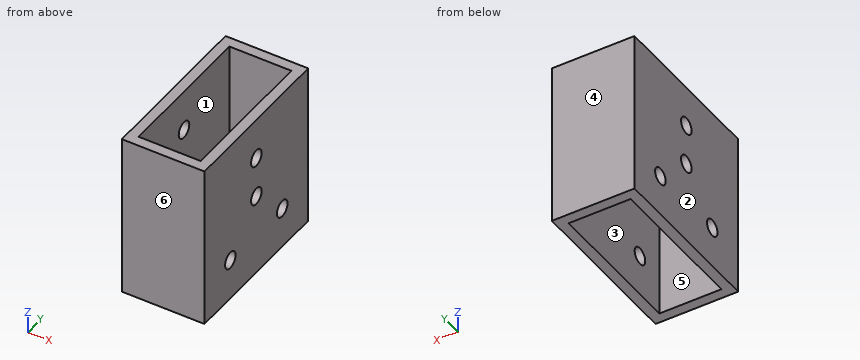
Autodesk Inventor part; units mm, degrees
ref_plane "YZ Plane" through (0, 0, 0) normal (1, 0, 0) x (0, 1, 0)
ref_plane "XZ Plane" through (0, 0, 0) normal (0, 1, 0) x (-1, 0, 0)
ref_plane "XY Plane" through (0, 0, 0) normal (0, 0, 1) x (1, 0, 0)
sketch "Sketch1" plane through (0, 0, 0) normal (0, 0, 1) x (1, 0, 0)
  line L0 (0, 0) -> (25.4, 0)
  line L1 (25.4, 0) -> (25.4, 50.8)
  line L2 (25.4, 50.8) -> (0, 50.8)
  line L3 (0, 50.8) -> (0, 0)
  line L4 (3.175, 47.625) -> (22.225, 47.625)
  line L5 (22.225, 47.625) -> (22.225, 3.175)
  line L6 (22.225, 3.175) -> (3.175, 3.175)
  line L7 (3.175, 3.175) -> (3.175, 47.625)
  dimension "d0" = 25.4
  dimension "d1" = 50.8
  dimension "d2" = 3.175
extrude "Extrusion1" add sketch "Sketch1" along normal blind 50.8
sketch "Sketch2" plane through (25.4, 0, 0) normal (1, 0, 0) x (0, 0, -1)
  line L0 (0, 50.8) -> (0, 0) construction
  line L1 (0, 0) -> (-12.7, 0) construction
  line L2 (0, 0) -> (-50.8, 0) construction
  line L3 (-12.7, 0) -> (-12.7, 12.7) construction
  line L4 (-12.7, 12.7) -> (-12.7, 38.1) construction
  circle A0 centre (-12.7, 12.7) radius 2.5797
  circle A1 centre (-12.7, 38.1) radius 2.5797
  dimension "d5" = 12.7
  dimension "d6" = 12.7
  dimension "d7" = 25.4
  dimension "d8" = 5.1594
extrude "Extrusion2" cut sketch "Sketch2" against normal blind 50.8
sketch "Sketch3" plane through (25.4, 0, 0) normal (1, 0, 0) x (0, 0, -1)
  line L0 (-50.8, 3.175) -> (-50.8, 47.625)
  line L1 (-50.8, 25.4) -> (-38.1, 25.4) construction
  line L2 (-38.1, 25.4) -> (-25.4, 25.4) construction
  circle A0 centre (-38.1, 25.4) radius 2.5797
  circle A1 centre (-25.4, 25.4) radius 2.5797
  point P0 (0, 0)
  dimension "d11" = 12.7
  dimension "d12" = 12.7
  dimension "d13" = 5.1594
extrude "Extrusion3" cut sketch "Sketch3" against normal blind 25.4
properties part number "2in 1x2"
CAD build for the part. Positions are in the model's coordinates, mm. Face numbers are marked on the shaded views. A direction names the side the tool comes from. Round coordinates to 2 decimals unless told otherwise and drop trailing zeros. Loops run counter-clockwise (first coordinate to the right, second up) from the corner with the lowest first, then second, coordinate; pieces in that order, holes last. Notation, with made-up numbers: M 9.25,-19 L 42.25,-19 A37 cw 42.25,17 Z; hole C 23.25,5.25 d6. An arc over 180 degrees is marked long. One line per question, with ' | ' between items. Start each with the question number.
Item 1: Cut at A-A, the plane z = 25.4. Write the cut outline in (x, y) (3 decimals).
Item 2: Cut at D-D, the plane y = 12.7. Write the cut outline in (x, z) (3 decimals), plus the area to 3 significant figures.
Item 3: Which spindle directions (+Z, -Z, +X, -X, +Y, -Y) get a long thin tool onto all of the face, cutting with end or side? Do the marked faces 5 and 6. Say none if no direction does.
Item 4: Two-plate mould, pull along X, no slides. Class the marked faces 1, 2, 3 and 4: pulls with the +X half, pulls with the -X half, needs draft (parallel to the pull), parting line crosses it, or undercut.
Item 5: Pin check, flat tip, straight feed: pin 1 Ø8.5 at (y, z) = (12.7, 12.7) entering from -X. Stop position of the tip, or through.
Item 6: Cut at C-C, the plane x = 2.5. Write the cut outline in (y, z), plus the area to 3 significant figures.
Item 7: Cut at B-B, the plane y = 22. Write the cut outline in (x, z) (3 decimals).
Item 8: Wall check: line 1 (Y direction, x = 2.4, z = 12.7); line 2 (X direction, y = 14, z = 38.5) (3 decimals); line 3 (Y direction, x = 13.75, z = 27) (3 decimals). Give the ranges that are in metal, low to high.
Responses:
1) outline: M 0,0 L 25.4,0 L 25.4,22.82 L 22.225,22.82 L 22.225,3.175 L 3.175,3.175 L 3.175,22.82 L 0,22.82 Z; M 0,27.98 L 3.175,27.98 L 3.175,47.625 L 22.225,47.625 L 22.225,27.98 L 25.4,27.98 L 25.4,50.8 L 0,50.8 Z
2) outline: M 0,0 L 3.175,0 L 3.175,10.12 L 0,10.12 Z; M 0,15.28 L 3.175,15.28 L 3.175,50.8 L 0,50.8 Z; M 22.225,0 L 25.4,0 L 25.4,10.12 L 22.225,10.12 Z; M 22.225,15.28 L 25.4,15.28 L 25.4,50.8 L 22.225,50.8 Z | area: 290 mm²
3) face 5: +Z, -Z | face 6: +Z, -Z, +X, -X, -Y
4) face 1: undercut | face 2: pulls with the -X half | face 3: undercut | face 4: needs draft
5) pin 1: stops at x = 0
6) outline: M 0,0 L 50.8,0 L 50.8,50.8 L 0,50.8 Z; hole C 12.7,12.7 d5.16; hole C 25.4,25.4 d5.16; hole C 25.4,38.1 d5.16; hole C 38.1,12.7 d5.16 | area: 2,500 mm²
7) outline: M 0,0 L 3.175,0 L 3.175,50.8 L 0,50.8 Z; M 22.225,0 L 25.4,0 L 25.4,50.8 L 22.225,50.8 Z
8) line 1: y = 0 to 10.12, 15.28 to 35.52, 40.68 to 50.8 | line 2: x = 0 to 3.175, 22.225 to 25.4 | line 3: y = 0 to 3.175, 47.625 to 50.8
